Source: CAD feature listing. Evaluate the final solid. Frame: model axes, mm. A direction names the side the tool comes from. Give positions to 0.01 mm unless a question says otherwise; leave off trailing zeros. Order: outer loops, then holes, each group sorted by start corner. A loop starts at its lowest first (then second) coordinate and runs counter-clockwise, first axis right, second up.
1) Draft query along Z for faces 1 (the face through (-6.85, 2, -6)), 2 (the face through (-5.36, 4.51, -6.23)), 3 (the face through (5, 2, 2)). Return one class per face: released by +Z, released by -Z, zero draft, split by the parting line, or undercut.
2) Access query for faces 4 (the face through (11, 0, -8)), 5 (the face through (0, 2, -2)), 6 (the face through (15.66, 4.51, -6.23)). Directions: +Z, -Z, +X, -X, +Y, -Y. A direction counts if a zero-diameter tool reaches every point of the face in a straight line with its end or side. Return the directions, or none.
3) Section D-D, the plane x = -1. Return loops of the section in (y, z).
4) Material intervals for line 1 (Z direction, x = 12.75, y = 1); line 2 (X direction, y = 3.8, z = -7.25); line 3 (X direction, y = 3.55, z = -11), sorted ascending.
5) First-contact query: P1, Ø2, axis at x = 4, z = -2.5, coming from the -Y side. Flat tip, straight axial feed; report the tip coordinate or a pass-through.
6) Section C-C, the plane z = -6. Return loops of the section in (x, y).
7) Section A-A, the plane x = 8.5. Return loops of the section in (y, z).
8) Section B-B, the plane y = 0.8. Return loops of the section in (x, z).
Autodesk Inventor part; units mm, degrees
ref_plane "YZ Plane" through (0, 0, 0) normal (1, 0, 0) x (0, 1, 0)
ref_plane "XZ Plane" through (0, 0, 0) normal (0, 1, 0) x (-1, 0, 0)
ref_plane "XY Plane" through (0, 0, 0) normal (0, 0, 1) x (1, 0, 0)
sketch "Sketch1" plane through (0, 0, 0) normal (0, 1, 0) x (-1, 0, 0)
  line L0 (0, 0) -> (-10.3, 0)
  line L1 (-10.3, 0) -> (-10.3, -12.5)
  line L2 (-10.3, -12.5) -> (0, -12.5)
  line L3 (0, -12.5) -> (0, 0)
  line L4 (6.85, -14.5) -> (-17.15, -14.5)
  line L5 (-17.15, -14.5) -> (-17.15, 2)
  line L6 (-17.15, 2) -> (6.85, 2)
  line L7 (6.85, 2) -> (6.85, -14.5)
  line L8 (0, -7.75) -> (4.85, -7.75)
  line L9 (4.85, -7.75) -> (4.85, -4.75)
  line L10 (4.85, -4.75) -> (0, -4.75)
  line L11 (-10.3, -7.75) -> (-15.15, -7.75)
  line L12 (-15.15, -7.75) -> (-15.15, -4.75)
  line L13 (-15.15, -4.75) -> (-10.3, -4.75)
  point P0 (-15.15, -6.25)
  point P1 (-10.3, -6.25)
  dimension "d0" = 3
  dimension "d1" = 10.3
  dimension "d2" = 12.5
  dimension "d3" = 2
  dimension "d4" = 2
  dimension "d5" = 2
  dimension "d6" = 2
  dimension "d7" = 20
extrude "Extrusion1" add sketch "Sketch1" along normal blind 5
chamfer "Chamfer1" distance 1 angle 45 2 edges at (-4.85, 5, -6.25) (15.15, 5, -6.25)
properties part number "Slot Detector Holder" material "ABS Plastic"
From the geometry:
1. face 1: zero draft
1. face 2: undercut
1. face 3: released by +Z
2. face 4: +Z, -Z, +X, -X, -Y
2. face 5: +Y, -Y
2. face 6: +Y
3. outline: (0, -14.5) - (5, -14.5) - (5, -7.75) - (0, -7.75) - close; (0, -4.75) - (5, -4.75) - (5, 2) - (0, 2) - close
4. line 1: z = -14.5 to -7.75, -4.75 to 2
4. line 2: x = -6.85 to -4.85, 15.15 to 17.15
4. line 3: x = -6.85 to 0, 10.3 to 17.15
5. P1: passes through
6. outline: (-6.85, 0) - (-4.85, 0) - (-4.85, 4) - (-5.85, 5) - (-6.85, 5) - close; (15.15, 0) - (17.15, 0) - (17.15, 5) - (16.15, 5) - (15.15, 4) - close
7. outline: (0, -14.5) - (5, -14.5) - (5, -12.5) - (0, -12.5) - close; (0, 0) - (5, 0) - (5, 2) - (0, 2) - close
8. outline: (-6.85, -14.5) - (17.15, -14.5) - (17.15, 2) - (-6.85, 2) - close; hole (-4.85, -7.75) - (0, -7.75) - (0, -12.5) - (10.3, -12.5) - (10.3, -7.75) - (15.15, -7.75) - (15.15, -4.75) - (10.3, -4.75) - (10.3, 0) - (0, 0) - (0, -4.75) - (-4.85, -4.75) - close
